from build123d import *

# Parameters (mm, degrees)
F0_W      = 76.2
F0_H      = 127
F1_DEPTH  = 25.4
F2_W      = 76.2
F2_H      = 25.4
F3_DEPTH  = 25.4
F4_W      = 58.42
F4_H      = 25.4
F5_DEPTH  = 25.4
F7_R      = 12.7
F8_DEPTH  = 25.4
F9_DEPTH  = 25.4
F10_DEPTH = 25.401


with BuildPart() as f1:
    # F0 (on Top) → F1 (new body)
    with BuildSketch(Plane.XY):
        with Locations((0.6532006686, 0.5051653504)):
            Rectangle(F0_W, F0_H)
    extrude(amount=F1_DEPTH)

    # F2 (on face) → F3 (join)
    with BuildSketch(Plane.XY.offset(25.4)):
        with Locations((0.6532006686, 51.3051653504)):
            Rectangle(F2_W, F2_H)
    extrude(amount=F3_DEPTH)

    # F4 (on face) → F5 (join)
    with BuildSketch(Plane.XY.offset(50.8)):
        with Locations((9.5432006686, 51.3051653504)):
            Rectangle(F4_W, F4_H)
    extrude(amount=F5_DEPTH)

    # F7 (on face) → F8 (cut)
    with BuildSketch(Plane.XY.offset(25.4)):
        with Locations((0, -28.8895512581)):
            Circle(F7_R)
    extrude(amount=-F8_DEPTH, mode=Mode.SUBTRACT)

    # F7 (on face) → F9 (cut)
    with BuildSketch(Plane.XY.offset(25.4)):
        with BuildLine():
            ThreePointArc((6.523787157, -62.3899730255), (-16.9822329005, -59.1992066955), (-35.3734492198, -44.2166457992))
            ThreePointArc((-35.3734492198, -44.2166457992), (-36.4439317634, -42.6534421545), (-37.4467993314, -41.0460233688))
            Line((-37.4467993314, -41.0460233688), (-37.4467993314, -62.9948346496))
            Line((-37.4467993314, -62.9948346496), (38.7532006686, -62.9948346496))
            Line((38.7532006686, -62.9948346496), (38.7532006686, -41.3434579968))
            ThreePointArc((38.7532006686, -41.3434579968), (25.0359793217, -55.5380857369), (6.523787157, -62.3899730255))
        make_face()
    extrude(amount=-F9_DEPTH, mode=Mode.SUBTRACT)

    # F7 (on face) → F10 (cut, through all)
    with BuildSketch(Plane.XY.offset(25.4)):
        with BuildLine():
            ThreePointArc((6.523787157, -62.3899730255), (-16.9822329005, -59.1992066955), (-35.3734492198, -44.2166457992))
            ThreePointArc((-35.3734492198, -44.2166457992), (-36.4439317634, -42.6534421545), (-37.4467993314, -41.0460233688))
            Line((-37.4467993314, -41.0460233688), (-37.4467993314, -62.9948346496))
            Line((-37.4467993314, -62.9948346496), (38.7532006686, -62.9948346496))
            Line((38.7532006686, -62.9948346496), (38.7532006686, -41.3434579968))
            ThreePointArc((38.7532006686, -41.3434579968), (25.0359793217, -55.5380857369), (6.523787157, -62.3899730255))
        make_face()
    extrude(amount=-F10_DEPTH, mode=Mode.SUBTRACT)


solid = f1.part
Input: part model. Units: mm. Frame: model coordinates. A direction names the side the tool comes from. Give positions to 0.01 mm unless a question says otherwise; leave off trailing zeros. Order: outer loops, then holes, each group sorted by start corner. A loop starts at its lowest first (then second) coordinate and runs counter-clockwise, first axis right, second up. Notation, with made-up numbers: (-23, 59) -> (14, 59) arc R10 ccw to (14, 70) -> close; hole circle Ø8 at (72.25, 73). An arc over 180 degrees is marked (long way). Use one line per item in the form item = value.
1) Section C-C, the plane z = 15.5. Return loops of the section in (x, y).
Response values:
outline = (-37.45, -41.05) arc R44.43 ccw to (-35.37, -44.22) arc R43.78 ccw to (6.52, -62.39) arc R44.43 ccw to (38.75, -41.34) -> (38.75, 64.01) -> (-37.45, 64.01) -> close; hole circle Ø25.4 at (0, -28.89)
2) Line query: probe 1 along Y at (x, z) = (0, 13.25); probe 2 along Z at (x, y) = (-22, -27.5); probe 3 along Y at (x, z) = (7.5, 7.5). Output: solid intervals per line, ascending.
Response values:
probe_1 = -62.81 to -41.59, -16.19 to 64.01
probe_2 = 0 to 25.4
probe_3 = -62.25 to -39.14, -18.64 to 64.01
3) Section B-B, the plane x = -3. Return loops of the section in (y, z), and give its area (3 significant figures).
Response values:
outline = (-62.68, 0) -> (-41.23, 0) -> (-41.23, 25.4) -> (-62.68, 25.4) -> close; (-16.55, 0) -> (64.01, 0) -> (64.01, 76.2) -> (38.61, 76.2) -> (38.61, 25.4) -> (-16.55, 25.4) -> close
area = 3,880 mm^2
4) Section D-D, the plane y = 47. Return loops of the section in (x, z), and give its area (3 significant figures).
Response values:
outline = (-37.45, 0) -> (38.75, 0) -> (38.75, 76.2) -> (-19.67, 76.2) -> (-19.67, 50.8) -> (-37.45, 50.8) -> close
area = 5,350 mm^2
5) Mould query, pull axis Y, two halves, no side actions, for faces 1 (the cylindrical face through (25.269, -55.385, 12.878)), 2 (the flat face through (0, 64.005, 38)), 3 (the cylindrical face through (-1.653, -16.298, 12.878)), 4 (the flat face through (-19.667, 51, 63)). Classes: pulls with the +Y half, pulls with the -Y half, needs draft (parallel to the pull), parting line crosses it, or undercut.
Response values:
face_1 = pulls with the -Y half
face_2 = pulls with the +Y half
face_3 = undercut
face_4 = needs draft
6) Reachability of faces 5 (the flat face through (-37.447, 22, 19)), 6 (the flat face through (0, 38.605, 50)), 7 (the flat face through (-29, 51, 50.8)) from +Z, -Z, +X, -X, +Y, -Y: full face, straight path, thin tool, end or side. Return the list, or none.
Response values:
face_5 = +Z, -Z, -X, +Y, -Y
face_6 = +Z, +X, -X, -Y
face_7 = +Z, -X, +Y, -Y
7) First-contact query: pin 1 Ø20.5 at (x, y) = (0, -28.89) entering from -Z; pin 2 Ø12 at (x, y) = (-27, 13) entering from +Z; pin 3 Ø9 at (x, y) = (-26, 57) entering from +Z; pin 4 Ø12 at (x, z) = (-24.5, 41) entering from -Y. Flat tips, straight axial feed; report the tip coordinate or a pass-through.
Response values:
pin_1 = through
pin_2 = 25.4
pin_3 = 50.8
pin_4 = 38.61
8) Section A-A, the plane y = -35. Return loops of the section in (x, z), and give its area (3 significant figures).
Response values:
outline = (-37.45, 0) -> (-11.13, 0) -> (-11.13, 25.4) -> (-37.45, 25.4) -> close; (11.13, 0) -> (38.75, 0) -> (38.75, 25.4) -> (11.13, 25.4) -> close
area = 1,370 mm^2
